Read the model definition and answer for the solid it produces. Units are mm, in the model's axes. A direction names the side the tool comes from. Round coordinates to 2 decimals unless told otherwise and drop trailing zeros. Loops run counter-clockwise (first coordinate to the right, second up) from the corner with the lowest first, then second, coordinate; pieces in that order, holes last. Notation, with made-up numbers: (-35, 43) - (23, 43) arc R9 cw to (23, 55) - close; hole circle Ø2 at (-2, 45.5). An arc over 180 degrees is marked (long way). Use CSV: the item, a comma, the result in double quotes. Start each with the question number.
1. Given pin 1 Ø4.5 at (x, y) = (0, 20) entering from +Z; pin 2 Ø2 at (x, y) = (0, 0) entering from -Z, each flat-ended and moving along its own axis, determine where each tip first touches the part or whether it passes through.
2. Find section A-A (y = -40). Give the vertices of the cut face in (x, z).
3. Find section B-B (z = 4.5). Give the vertices of the cut face in (x, y), and give its area (3 significant figures).
4. Find section C-C (y = 9.5). Give the vertices of the cut face in (x, z), and give its area (3 significant figures).
5. Consider line 1 along X through (y, z) = (0, 5.95); line 2 along X through (y, z) = (-40, 1.8); line 3 along Z through (x, y) = (-1.25, 22). Determine where each line is inside the solid, lowest interval first.
6. A tool of negligible diameter and unlimited length cuts with its end or side. For faces 4 (the cylindrical face through (-0.08, 21.85, 1.7)), 5 (the flat face through (1, 2, 3.44)), from which of +Z, -Z, +X, -X, +Y, -Y can it reach the whole face along a straight path? Write none if from no direction.
7. Determine the mould class of faces 1 (the cylindrical face through (1.168, 42.817, 4.991)), 2 (the cylindrical face through (-3.5, -0.7, 4.5)), 3 (the flat face through (4.5, -1, 2)) for opening direction X: +X half, -X half, draft (parallel to the pull), parting line (faces both ways), or undercut.
from build123d import *

# Parameters (mm, degrees)
PAD_DEPTH           = 50
CHAMFER003_SIZE     = 0.35
HOLE001_D           = 3.7
HOLE001_CBORE_D     = 6.1
HOLE001_CBORE_DEPTH = 3.06


with BuildPart() as part:
    # Sketch → Pad (new body, symmetric)
    with BuildSketch(Plane.XZ):
        with BuildLine():
            Line((-4.5, 6.5), (4.5, 6.5))
            Line((4.5, 6.5), (4.5, 5.5))
            ThreePointArc((4.5, 5.5), (3.5, 4.5), (4.5, 3.5))
            Line((4.5, 3.5), (4.5, 0))
            Line((4.5, 0), (-4.5, 0))
            Line((-4.5, 0), (-4.5, 3.5))
            ThreePointArc((-4.5, 3.5), (-3.5, 4.5), (-4.5, 5.5))
            Line((-4.5, 5.5), (-4.5, 6.5))
        make_face()
    extrude(amount=PAD_DEPTH, both=True)

    # Chamfer003
    chamfer003_edges = [part.edges().sort_by_distance(p)[0] for p in [
        (4.5, 0, 6.5),
        (4.5, 0, 0),
        (-4.5, 0, 0),
        (-4.5, 0, 6.5),
    ]]
    chamfer(chamfer003_edges, length=CHAMFER003_SIZE)

    # Hole001 (through all)
    with Locations(Plane(origin=(0, 0, 6.5), x_dir=(0, 1, 0), z_dir=(0, 0, 1))):
        with Locations((0, 0), (-20, 0), (-40, 0), (-60, 0), (-80, 0), (-100, 0), (-120, 0), (-140, 0), (-160, 0), (-180, 0), (20, 0), (40, 0), (60, 0), (80, 0), (100, 0), (120, 0), (140, 0), (160, 0), (180, 0)):
            CounterBoreHole(HOLE001_D / 2, HOLE001_CBORE_D / 2, HOLE001_CBORE_DEPTH)


solid = part.part
Filled sheet:
1,pin 1,"stops at z = 3.44"
1,pin 2,"passes through"
2,outline,"(-4.5, 0.35) - (-4.15, 0) - (-1.85, 0) - (-1.85, 3.44) - (-3.05, 3.44) - (-3.05, 6.5) - (-4.15, 6.5) - (-4.5, 6.15) - (-4.5, 5.5) arc R1 cw to (-4.5, 3.5) - close; (1.85, 0) - (4.15, 0) - (4.5, 0.35) - (4.5, 3.5) arc R1 cw to (4.5, 5.5) - (4.5, 6.15) - (4.15, 6.5) - (3.05, 6.5) - (3.05, 3.44) - (1.85, 3.44) - close"
3,outline,"(-3.5, -50) - (3.5, -50) - (3.5, 50) - (-3.5, 50) - close; hole circle Ø6.1 at (0, -40); hole circle Ø6.1 at (0, -20); hole circle Ø6.1 at (0, 0); hole circle Ø6.1 at (0, 20); hole circle Ø6.1 at (0, 40)"
3,area,"554 mm²"
4,outline,"(-4.5, 0.35) - (-4.15, 0) - (4.15, 0) - (4.5, 0.35) - (4.5, 3.5) arc R1 cw to (4.5, 5.5) - (4.5, 6.15) - (4.15, 6.5) - (-4.15, 6.5) - (-4.5, 6.15) - (-4.5, 5.5) arc R1 cw to (-4.5, 3.5) - close"
4,area,"55.1 mm²"
5,line 1,"x = -4.5 to -3.05, 3.05 to 4.5"
5,line 2,"x = -4.5 to -1.85, 1.85 to 4.5"
5,line 3,"z = 0 to 3.44"
6,face 4,"+Z, -Z"
6,face 5,"+Z"
7,face 1,"undercut"
7,face 2,"-X half"
7,face 3,"+X half"
